Read the model definition and answer for the solid it produces. Units are mm, in the model's axes. A direction names the side the tool comes from. Give positions to 0.01 mm unless a question says otherwise; leave off trailing zeros. Loops run counter-clockwise (first coordinate to the right, second up) from the corner with the lowest first, then second, coordinate; pieces in that order, holes last. Notation, with made-up numbers: (47, -22.75) - (105, -22.75) arc R27 ccw to (105, -2.75) - close; hole circle Ø1 at (25, 71.25). An arc over 180 degrees is marked (long way). Write each question's results on one line, items separated by ' | '. Start each with the question number.
Q1. For faces 1 (the flat face through (0, 0, 34)), 2 (the cylindrical face through (-7.493, -0.33, 26.395)), 3 (the flat face through (4, 7, -19)), determine the directions among +Z, -Z, +X, -X, +Y, -Y from which every point of the face is accessible in a straight line to the end or side of a thin tool.
Q2. Find the intervals of material crossed by line 1 (Z direction, x = -7, y = 3.5); line 2 (Y direction, x = 0.25, z = -13); line 3 (X direction, y = -2, z = 29.5), in increasing order. Write a range as from..to.
Q3. The part is cut by section D-D, the plane z = -4. Write down the section's boundary in (x, y).
Q4. The part is cut by section A-A, the plane x = 0. Write down the section's boundary in (y, z).
Q5. The part is cut by section C-C, the plane z = -24. Write down the section's boundary in (x, y).
Q6. Given pin 1 (2 mm diameter, centred on y = -2.5, z = -25.5, fed in from -X); pin 2 (12 mm diameter, centred on x = -5.5, z = 11, fed in from +Y); pin 3 (10 mm diameter, centred on y = -7, z = 6, fed in from -X); pin 4 (4 mm diameter, centred on x = 5.5, z = 2, fed in from -Y), each flat-ended and moving along its own axis, determine where each tip first touches the part or whether it passes through.
Autodesk Inventor part; units mm, degrees
ref_plane "YZ Plane" through (0, 0, 0) normal (1, 0, 0) x (0, 1, 0)
ref_plane "XZ Plane" through (0, 0, 0) normal (0, 1, 0) x (-1, 0, 0)
ref_plane "XY Plane" through (0, 0, 0) normal (0, 0, 1) x (1, 0, 0)
sketch "Sketch1" plane through (0, 0, 0) normal (0, 0, 1) x (1, 0, 0)
  circle A0 centre (0, 0) radius 10
  dimension "d0" = 20
extrude "Extrusion1" add sketch "Sketch1" along normal mid plane 38
sketch "Sketch2" plane through (0, 0, 19) normal (0, 0, 1) x (1, 0, 0)
  circle A0 centre (0, 0) radius 7.5
  dimension "d3" = 15
extrude "Extrusion2" add sketch "Sketch2" along normal blind 15
sketch "Sketch3" plane through (0, 0, -19) normal (0, 0, -1) x (-1, 0, 0)
  circle A0 centre (0, 0) radius 7.5
  dimension "d7" = 15
extrude "Extrusion3" add sketch "Sketch3" along normal blind 30
equation "\"d7\" = d3"
properties part number "Foreas_1"
Check sheet entries:
1) face 1: +Z, +X, -X, +Y, -Y | face 2: +Z | face 3: -Z
2) line 1: z = -19..19 | line 2: y = -10..10 | line 3: x = -7.23..7.23
3) outline: circle Ø20 at (0, 0)
4) outline: (-10, -19) - (-7.5, -19) - (-7.5, -49) - (7.5, -49) - (7.5, -19) - (10, -19) - (10, 19) - (7.5, 19) - (7.5, 34) - (-7.5, 34) - (-7.5, 19) - (-10, 19) - close
5) outline: circle Ø15 at (0, 0)
6) pin 1: stops at x = -7.35 | pin 2: stops at y = 10 | pin 3: stops at x = -9.8 | pin 4: stops at y = -9.37
